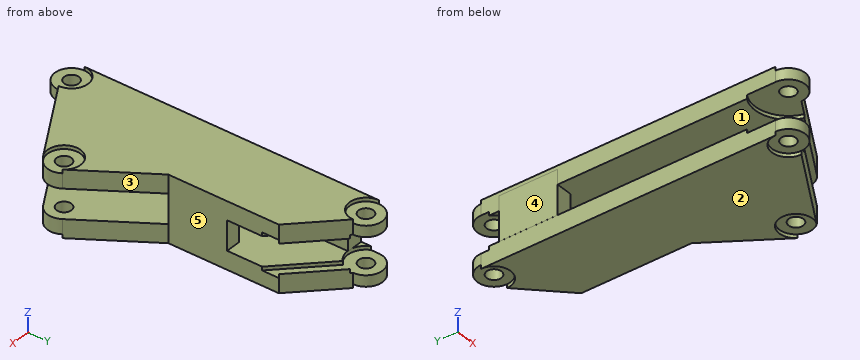
Autodesk Inventor part; units mm, degrees
ref_plane "Work Plane1" through (0, 0, 2) normal (0, 0, 1) x (1, 0, 0)
ref_plane "Work Plane2" through (0, 0, 2) normal (0, 0, -1) x (-1, 0, 0)
ref_plane "YZ Plane" through (0, 0, 0) normal (1, 0, 0) x (0, 1, 0)
sketch "Sketch1" plane through (0, 0, 0) normal (0, 0, 1) x (1, 0, 0)
  circle A0 centre (0, 0) radius 1
  circle A1 centre (0, 0) radius 2.25
  circle A2 centre (0, 40) radius 1
  circle A3 centre (0, 40) radius 2.25
  line L0 (-2.25, 40) -> (-2.25, 0)
  line L1 (0, 0) -> (15, 0) construction
  line L2 (12.2873, 8.6036) -> (11.2873, 8.6036)
  circle A4 centre (12.2873, 8.6036) radius 1
  circle A5 centre (12.2873, 8.6036) radius 2.25
  line L3 (2.25, 0) -> (13.4395, 6.671)
  line L4 (2.25, 40) -> (7.9069, 34.3431)
  line L5 (7.9069, 34.3431) -> (7.9069, 19.3431)
  line L6 (7.9069, 19.3431) -> (14.1662, 9.8414)
  line L7 (0, 0) -> (0, 1)
  line L8 (0, 39) -> (0, 40)
  line L9 (0, 0) -> (1.8431, 1.2905)
  line L10 (11.4681, 8.0301) -> (12.2873, 8.6036)
  dimension "d5" = 2
  dimension "d7" = 2
  dimension "d0" = 40
  dimension "d6" = 4.5
  dimension "d8" = 4.5
  dimension "d9" = 15
  dimension "d11" = 2
  dimension "d12" = 4.5
  dimension "d13" = 8
  dimension "d15" = 15
ref_plane "Work Plane1" through (0, 0, 2) normal (0, 0, 1) x (1, 0, 0)
extrude "Extrusion1" add sketch "Sketch1" against normal blind 2.5 contours A1 L0 A3 L4 L5 L6 A5 L3
extrude "Extrusion2" add sketch "Sketch1" against normal blind 2 contours A1 | A5 | A3
mirror "Mirror1" about plane through (0, 0, 2) normal (0, 0, 1) of "Extrusion1", "Extrusion2"
sketch "Sketch2" plane through (0, 0, 0) normal (0, 0, 1) x (1, 0, 0)
  line L0 (0, 37.5855) -> (-2.2556, 37.5855)
  line L1 (-2.2556, 37.5855) -> (-2.2556, 29.5855)
  line L2 (-2.2556, 29.5855) -> (0, 29.5855)
  line L3 (0, 29.5855) -> (0, 37.5855)
  point P0 (0, 0)
  dimension "d21" = 8
extrude "Extrusion3" add sketch "Sketch2" along normal blind 6
sketch "Sketch3" plane through (0, 0, 6.5) normal (0, 0, 1) x (1, 0, 0)
  line L0 (7.9069, 19.3431) -> (5.9069, 19.3431)
  line L1 (5.9069, 19.3431) -> (5.9069, 27.3431)
  line L2 (5.9069, 27.3431) -> (7.9069, 27.3431)
  line L3 (7.9069, 27.3431) -> (7.9069, 19.3431)
  point P0 (0, 0)
  dimension "d24" = 2
  dimension "d25" = 8
extrude "Extrusion4" add sketch "Sketch3" against normal blind 9
sketch "Sketch6" plane through (0, 0, 4) normal (0, 0, -1) x (-1, 0, 0)
  circle A0 centre (0, 0) radius 4.5
  dimension "d33" = 9
extrude "Extrusion7" cut sketch "Sketch6" against normal blind 0.5
sketch "Sketch7" plane through (0, 0, 0) normal (0, 0, 1) x (1, 0, 0)
  circle A0 centre (0, 0) radius 4.5
  dimension "d36" = 9
extrude "Extrusion8" cut sketch "Sketch7" against normal blind 0.5
sketch "Sketch8" plane through (0, 40, 4) normal (0, 0, -1) x (-1, 0, 0)
  circle A0 centre (0, 0) radius 2.5
  line L0 (-1.7678, -1.7678) -> (-6.7819, -6.7819)
  circle A1 centre (0, 0) radius 2.5
  line L1 (-7.9069, -5.6569) -> (-2.4944, -0.2556)
  arc A2 (-2.4876, -0.2488) -> (-1.7678, -1.7678) centre (0, 0) ccw
  arc A3 (-2.4876, -0.2488) -> (-1.7678, -1.7678) centre (0, 0) ccw
  line L2 (-7.9069, -5.6569) -> (-2.4876, -0.2488)
  line L3 (-7.9069, -5.6569) -> (-7.9069, -7.9069)
  line L4 (-6.7819, -6.7819) -> (-7.9069, -7.9069)
  point P0 (0, -40)
  dimension "d39" = 5
extrude "Extrusion9" cut sketch "Sketch8" against normal blind 0.5
ref_plane "Work Plane2" through (0, 0, 2) normal (0, 0, -1) x (-1, 0, 0)
mirror "Mirror2" about plane through (0, 0, 2) normal (0, 0, -1) of "Extrusion9"
properties part number "Pinky_Lower_main_1"
Can you work these out from the model? Positions are in its coordinate system, mm. Face numbers are marked on the shaded views. A direction names the side the tool comes from. Round coordinates to 2 decimals unless told otherwise and drop trailing zeros. Order: outer loops, then holes, each group sorted by start corner. A loop starts at its lowest first (then second) coordinate and runs counter-clockwise, first axis right, second up. Notation, with made-up numbers: M 50,46 L 96,46 A7 ccw 96,57 Z; hole C -4.5,78.5 d5. An arc over 180 degrees is marked long. Use a Markdown table: item, result.
1) If we mould it in two halves opening along Z, with no side actions, what happens to the marked faces 1, 2 and 3? For each: +Z half, -Z half, draft (parallel to the pull), parting line (faces both ways), or undercut.
Geometry says:
| item | result |
|---|---|
| face 1 | undercut |
| face 2 | -Z half |
| face 3 | draft |
2) Imagine slicing it at A-A (z = 1.5). List the corners of the cut face in (x, y) for me, then the cut area to 3 significant figures.
Geometry says:
| item | result |
|---|---|
| outline | M -2.26,29.59 L 0,29.59 L 0,37.59 L -2.26,37.59 Z; M 5.91,19.34 L 7.91,19.34 L 7.91,27.34 L 5.91,27.34 Z |
| area | 34.0 mm² |
3) If I drill on line 1 along Y through (x, z) = (0, 5.35); line 2 along Z through (x, y) = (6.75, 32.5); line 3 along Z through (x, y) = (7, 34.5), over which ranges is the centre line in solid material (lowest first)?
Geometry says:
| item | result |
|---|---|
| line 1 | y = -2.25 to -1, 1 to 39, 41 to 42.25 |
| line 2 | z = -2.5 to 0, 4 to 6.5 |
| line 3 | z = -2.5 to -0.5, 4.5 to 6.5 |
4) I'm going to push flat-ended pins straight in: P1, Ø1, axis at y = 33, z = 5, coming from the +X side; P2, Ø3, axis at x = 0, y = 40, coming from the +Z side; P3, Ø1.2, axis at y = 32.5, z = 2, coming from the +X side. Where does each tip first touch, or does it pass through?
Geometry says:
| item | result |
|---|---|
| P1 | stops at x = 7.91 |
| P2 | stops at z = 6 |
| P3 | stops at x = 0 |
5) On a 3-axis mill with a long thin cutter (end or side, diameter ignored), from which of +Z, -Z, +X, -X, +Y, -Y can I reach the whole of each face in a straight line? I mean the marked faces 4 and 5. Say none if no direction works.
Geometry says:
| item | result |
|---|---|
| face 4 | +Z, -Z, -X, +Y, -Y |
| face 5 | +Z, -Z, +X, +Y |
6) Imagine slicing it at B-B (x = 9). List the corners of the cut face in (y, z) for me, then the cut area to 3 significant figures.
Geometry says:
| item | result |
|---|---|
| outline | M 4.02,-2.5 L 17.68,-2.5 L 17.68,0 L 4.02,0 Z; M 4.02,4 L 17.68,4 L 17.68,6.5 L 4.02,6.5 Z |
| area | 68.3 mm² |
